```python
from build123d import *

# Parameters (mm, degrees)
CYLINDER_R     = 1.6
CYLINDER_DEPTH = 10
BOX_W          = 10
BOX_H          = 10
BOX_DEPTH      = 2


with BuildPart() as cylinder:
    # Cylinder → Cylinder (new body)
    with BuildSketch(Plane(origin=(5, 5, -4), x_dir=(1, 0, 0), z_dir=(0, 0, 1))):
        Circle(CYLINDER_R)
    extrude(amount=CYLINDER_DEPTH)


with BuildPart() as cut:
    # Box → Box (new body)
    with BuildSketch(Plane.XY):
        with Locations((5, 5)):
            Rectangle(BOX_W, BOX_H)
    extrude(amount=BOX_DEPTH)

    # Cut: cut Cylinder
    add(cylinder.part, mode=Mode.SUBTRACT)


solid = cut.part
```
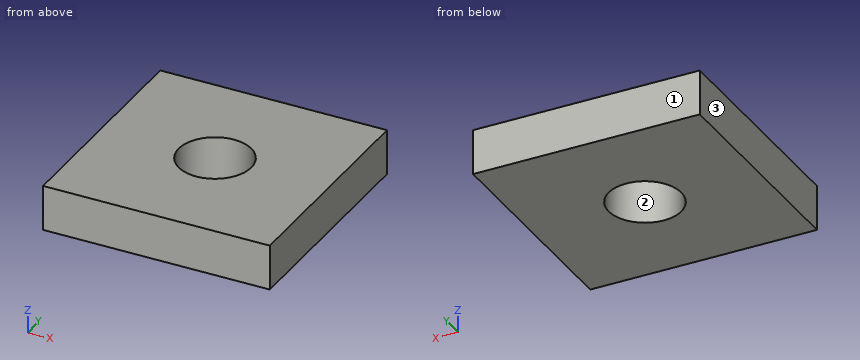
CAD build for the part. Positions are in the model's coordinates, mm. Face numbers are marked on the shaded views. Give positions to 0.01 mm unless a question says otherwise; leave off trailing zeros. Loops run counter-clockwise (first coordinate to the right, second up) from the corner with the lowest first, then second, coordinate; pieces in that order, holes last. Notation, with made-up numbers: (5, 33) - (19, 33) arc R20 ccw to (19, 68) - close; hole circle Ø4 at (79, 44). An arc over 180 degrees is marked (long way). Put each result on its own line as item: value.
Q1. Flat gauge pin, fed straight in: pin 1 (3 mm diameter, centred on x = 5, y = 5, fed in from +Z). Where does the tip first touch, or does it go through?
Filled in:
pin 1: passes through
Q2. Mould opens along Y. For the marked faces 1, 2 and 3 say: pulls with the +Y half, pulls with the -Y half, needs draft (parallel to the pull), parting line crosses it, or undercut.
Filled in:
face 1: pulls with the +Y half
face 2: undercut
face 3: needs draft
Q3. Slice it at A-A (y = 5). Give the cut face in (x, z), plus the area to 3 significant figures.
Filled in:
outline: (0, 0) - (3.4, 0) - (3.4, 2) - (0, 2) - close; (6.6, 0) - (10, 0) - (10, 2) - (6.6, 2) - close
area: 13.6 mm²
Q4. Slice it at C-C (z = 1). Give the cut face in (x, y).
Filled in:
outline: (0, 0) - (10, 0) - (10, 10) - (0, 10) - close; hole circle Ø3.2 at (5, 5)
Q5. Probe line 1 along X through (y, z) = (5, 1.3); line 2 along Y through (x, z) = (4, 0.2). List the from-to ranges inside material, lowest first.
Filled in:
line 1: x = 0 to 3.4, 6.6 to 10
line 2: y = 0 to 3.75, 6.25 to 10
